```python
from build123d import *

# Parameters (mm, degrees)
SKETCH1_W           = 25.4
SKETCH1_H           = 50.8
SKETCH1_W_2         = 19.05
SKETCH1_H_2         = 44.45
BOSS_EXTRUDE1_DEPTH = 914.4
SKETCH2_R           = 2.4892
CUT_EXTRUDE1_DEPTH  = 916.898078391


with BuildPart() as part:
    # Sketch1 → Boss-Extrude1 (new body)
    with BuildSketch(Plane.XY):
        Rectangle(SKETCH1_W, SKETCH1_H)
        Rectangle(SKETCH1_W_2, SKETCH1_H_2, mode=Mode.SUBTRACT)
    extrude(amount=BOSS_EXTRUDE1_DEPTH)

    # Sketch2 → Cut-Extrude1 (cut, through all)
    with BuildSketch(Plane(origin=(0, 25.4, 0), x_dir=(1, 0, 0), z_dir=(0, 1, 0))):
        with Locations(Location((0, -12.7, 0), (0, 0, 270))):
            Circle(SKETCH2_R)
        with Locations(Location((0, -25.4, 0), (0, 0, 270))):
            Circle(SKETCH2_R)
        with Locations(Location((0, -38.1, 0), (0, 0, 270))):
            Circle(SKETCH2_R)
        with Locations(Location((0, -50.8, 0), (0, 0, 270))):
            Circle(SKETCH2_R)
        with Locations(Location((0, -63.5, 0), (0, 0, 270))):
            Circle(SKETCH2_R)
        with Locations(Location((0, -76.2, 0), (0, 0, 270))):
            Circle(SKETCH2_R)
        with Locations(Location((0, -88.9, 0), (0, 0, 270))):
            Circle(SKETCH2_R)
        with Locations(Location((0, -101.6, 0), (0, 0, 270))):
            Circle(SKETCH2_R)
    extrude(amount=-CUT_EXTRUDE1_DEPTH, mode=Mode.SUBTRACT)


solid = part.part
```
Design review of the part built by this model. Coordinates are the model's own, in mm. A direction names the side the tool comes from. Give positions to 0.01 mm unless a question says otherwise; leave off trailing zeros. Write each loop counter-clockwise with the first axis right and the second up, starting at its lowest first coordinate (ties: lowest second). Pieces come first, ordered by that corner, then holes. Notation, with made-up numbers: (72, -35.75) -> (95, -35.75) arc R8 ccw to (95, -26.75) -> close; hole circle Ø7 at (-23, 75.5). An arc over 180 degrees is marked (long way). Answer in a Markdown table with one row per item.
(1) To check wall thickness, follow probe 1 along Y at (x, z) = (-5.75, 310.5) (3 decimals); probe 2 along X at (y, z) = (-2, 821) (3 decimals); probe 3 along X at (y, z) = (-23.8, 12.7). State the ranges of each line that lie inside material, in increasing order.
Results:
| item | result |
|---|---|
| probe 1 | -25.4 to -22.225, 22.225 to 25.4 |
| probe 2 | -12.7 to -9.525, 9.525 to 12.7 |
| probe 3 | -12.7 to -2.49, 2.49 to 12.7 |
(2) For faces 4 (the flat face through (0, -22.225, 451)), 5 (the flat face through (-10, -2, 0)), list the 3-axis set-ups (+Z, -Z, +X, -X, +Y, -Y) from which the entire face can be reached by the end or side of a thin tool; tool diameter is ignored.
Results:
| item | result |
|---|---|
| face 4 | +Z, -Z |
| face 5 | -Z, +X, -X, +Y, -Y |
(3) Consider section B-B (y = 10.5). State the section outline as (x, z) points (3 decimals), then the cut area to 3 significant figures.
Results:
| item | result |
|---|---|
| outline | (-12.7, 0) -> (-9.525, 0) -> (-9.525, 914.4) -> (-12.7, 914.4) -> close; (9.525, 0) -> (12.7, 0) -> (12.7, 914.4) -> (9.525, 914.4) -> close |
| area | 5,810 mm2 |
(4) Consider section A-A (z = 487). State the section outline as (x, y) points (3 decimals), then the cut area to 3 significant figures.
Results:
| item | result |
|---|---|
| outline | (-12.7, -25.4) -> (12.7, -25.4) -> (12.7, 25.4) -> (-12.7, 25.4) -> close; hole (-9.525, -22.225) -> (9.525, -22.225) -> (9.525, 22.225) -> (-9.525, 22.225) -> close |
| area | 444 mm2 |
(5) Mouldability with a two-part tool opening along X and no side actions: class faces 1 (the flat face through (0, -25.4, 451)), 2 (the flat face through (12.7, 0, 451)), 3 (the flat face through (0, 22.225, 451)) as +X half, -X half, draft (parallel to the pull), parting line (faces both ways), or undercut.
Results:
| item | result |
|---|---|
| face 1 | draft |
| face 2 | +X half |
| face 3 | undercut |
(6) Clearance check with a flat-ended pin moving along its axis: pin 1 (4 mm diameter, centred on x = 0, z = 88.9, fed in from -Y). State where the tip first meets the part, or that it passes through.
Results:
| item | result |
|---|---|
| pin 1 | through |
